from build123d import *

# Parameters (mm, degrees)
SKETCH1_W                 = 350
SKETCH1_H                 = 300
BOSS_EXTRUDE1_DEPTH       = 6.35
SKETCH2_R                 = 4.25
CUT_EXTRUDE1_DEPTH        = 7.35
LPATTERN2_COUNT           = 2
LPATTERN2_PITCH           = 200
LPATTERN3_COUNT           = 2
LPATTERN3_PITCH           = 250
LPATTERN3_COPY_1_SKETCH_R = 4.25
LPATTERN3_COPY_1_DEPTH    = 7.35
FILLET1_R                 = 10
SKETCH4_R                 = 1.75
CUT_EXTRUDE2_DEPTH        = 7.35
LPATTERN5_COUNT           = 2
LPATTERN5_PITCH           = 80
LPATTERN5_COUNT_DIR2      = 2
LPATTERN5_PITCH_DIR2      = 80
SKETCH5_R                 = 1.75
CUT_EXTRUDE3_DEPTH        = 7.35
LPATTERN6_COUNT           = 2
LPATTERN6_PITCH           = 22.23
LPATTERN6_COUNT_DIR2      = 2
LPATTERN6_PITCH_DIR2      = 135
SKETCH7_R                 = 1.75
CUT_EXTRUDE4_DEPTH        = 7.35
LPATTERN9_COUNT           = 2
LPATTERN9_PITCH           = 22.23
LPATTERN9_COUNT_DIR2      = 2
LPATTERN9_PITCH_DIR2      = 135


with BuildPart() as part:
    # Sketch1 → Boss-Extrude1 (new body)
    with BuildSketch(Plane(origin=(0, 0, 0), x_dir=(1, 0, 0), z_dir=(0, 1, 0))):
        Rectangle(SKETCH1_W, SKETCH1_H)
    extrude(amount=BOSS_EXTRUDE1_DEPTH)

    # Sketch2 → Cut-Extrude1 (cut, through all)
    with BuildSketch(Plane.XZ):
        with Locations((-125, -100)):
            Circle(SKETCH2_R)
    cut_extrude1 = extrude(amount=-CUT_EXTRUDE1_DEPTH, mode=Mode.SUBTRACT)

    # LPattern2: Cut-Extrude1 ×2
    with Locations(*[(0, 0, i * LPATTERN2_PITCH) for i in range(1, LPATTERN2_COUNT)]):
        add(cut_extrude1, mode=Mode.SUBTRACT)

    # LPattern3: Cut-Extrude1 ×2
    with Locations(*[(i * LPATTERN3_PITCH, 0, 0) for i in range(1, LPATTERN3_COUNT)]):
        add(cut_extrude1, mode=Mode.SUBTRACT)

    # LPattern3 copy 1 sketch → LPattern3 copy 1 (cut, through all)
    with BuildSketch(Plane(origin=(250, 0, 200), x_dir=(1, 0, 0), z_dir=(0, -1, 0))):
        with Locations((-125, -100)):
            Circle(LPATTERN3_COPY_1_SKETCH_R)
    extrude(amount=-LPATTERN3_COPY_1_DEPTH, mode=Mode.SUBTRACT)

    # Fillet1
    fillet1_edges = [part.edges().sort_by_distance(p)[0] for p in [
        (-175, 3.175, -150),
        (175, 3.175, -150),
        (175, 3.175, 150),
        (-175, 3.175, 150),
    ]]
    fillet(fillet1_edges, radius=FILLET1_R)

    # Sketch4 → Cut-Extrude2 (cut, through all)
    with BuildSketch(Plane.XZ):
        Circle(SKETCH4_R)
    cut_extrude2 = extrude(amount=-CUT_EXTRUDE2_DEPTH, mode=Mode.SUBTRACT)

    # LPattern5: Cut-Extrude2 2 × 2
    with Locations(*[(i * LPATTERN5_PITCH, 0, j * LPATTERN5_PITCH_DIR2) for i in range(LPATTERN5_COUNT) for j in range(LPATTERN5_COUNT_DIR2) if (i, j) != (0, 0)]):
        add(cut_extrude2, mode=Mode.SUBTRACT)

    # Sketch5 → Cut-Extrude3 (cut, through all)
    with BuildSketch(Plane.XZ):
        with Locations((-141.82, -67.5)):
            Circle(SKETCH5_R)
    cut_extrude3 = extrude(amount=-CUT_EXTRUDE3_DEPTH, mode=Mode.SUBTRACT)

    # LPattern6: Cut-Extrude3 2 × 2
    with Locations(*[(-i * LPATTERN6_PITCH, 0, j * LPATTERN6_PITCH_DIR2) for i in range(LPATTERN6_COUNT) for j in range(LPATTERN6_COUNT_DIR2) if (i, j) != (0, 0)]):
        add(cut_extrude3, mode=Mode.SUBTRACT)

    # Sketch7 → Cut-Extrude4 (cut, through all)
    with BuildSketch(Plane.XZ):
        with Locations((141.82, -67.5)):
            Circle(SKETCH7_R)
    cut_extrude4 = extrude(amount=-CUT_EXTRUDE4_DEPTH, mode=Mode.SUBTRACT)

    # LPattern9: Cut-Extrude4 2 × 2
    with Locations(*[(i * LPATTERN9_PITCH, 0, j * LPATTERN9_PITCH_DIR2) for i in range(LPATTERN9_COUNT) for j in range(LPATTERN9_COUNT_DIR2) if (i, j) != (0, 0)]):
        add(cut_extrude4, mode=Mode.SUBTRACT)


solid = part.part
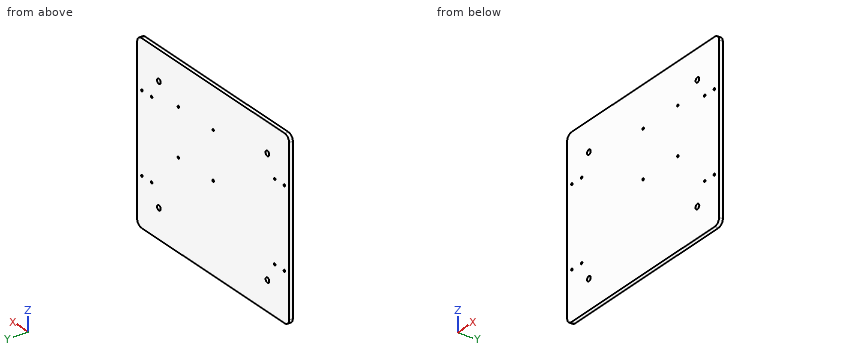
Could you check a few things on this model? Use its own coordinates, in mm. Round coordinates to 2 decimals unless told otherwise and drop trailing zeros. Write each loop counter-clockwise with the first axis right and the second up, starting at its lowest first coordinate (ties: lowest second). Pieces come first, ordered by that corner, then holes. Notation, with made-up numbers: (26.25, -20.75) - (54.25, -20.75) arc R24 ccw to (54.25, 11.25) - close; hole circle Ø9 at (-19.75, 89). An arc over 180 degrees is marked (long way). Put each result on its own line as item: value. Start each with the question number.
(1) I want a section at A-A, the plane x = 125. Please give me the cut outline in (y, z), plus the area to 3 significant figures.
(2) I want a section at B-B, the plane z = 100. Please give me the cut outline in (x, y), plus the area to 3 significant figures.
(3) I need wall thicknesses on probe 1 along X at (y, z) = (4.5, 67.5); probe 2 along Z at (x, y) = (125, 2.5); probe 3 along Z at (x, y) = (164.05, 1.75). Which ranges of each line are inside material? Lowest first, please.
(4) Will these pins go through, and if not, where does the flat tip stop? pin 1 (3 mm diameter, centred on x = -141.82, z = 67.5, fed in from +Y); pin 2 (12 mm diameter, centred on x = 122, z = -28.5, fed in from -Y).
Here are the results:
1. outline: (0, -150) - (6.35, -150) - (6.35, -104.25) - (0, -104.25) - close; (0, -95.75) - (6.35, -95.75) - (6.35, 95.75) - (0, 95.75) - close; (0, 104.25) - (6.35, 104.25) - (6.35, 150) - (0, 150) - close
1. area: 1,800 mm^2
2. outline: (-175, 0) - (-129.25, 0) - (-129.25, 6.35) - (-175, 6.35) - close; (-120.75, 0) - (120.75, 0) - (120.75, 6.35) - (-120.75, 6.35) - close; (129.25, 0) - (175, 0) - (175, 6.35) - (129.25, 6.35) - close
2. area: 2,110 mm^2
3. probe 1: x = -175 to -165.8, -162.3 to -143.57, -140.07 to 140.07, 143.57 to 162.3, 165.8 to 175
3. probe 2: z = -150 to -104.25, -95.75 to 95.75, 104.25 to 150
3. probe 3: z = -150 to -69.25, -65.75 to 65.75, 69.25 to 150
4. pin 1: passes through
4. pin 2: stops at y = 0
